Read the model definition and answer for the solid it produces. Units are mm, in the model's axes. A direction names the side the tool comes from. Coordinates: 2 decimals unless noted, no trailing zeros. Write each loop counter-clockwise with the first axis right and the second up, starting at its lowest first coordinate (ties: lowest second). Pieces come first, ordered by that corner, then holes. Notation, with made-up numbers: (18.25, 38.25) - (39.25, 38.25) arc R8 cw to (39.25, 47.25) - close; hole circle Ø9 at (-6.75, 79). An arc over 180 degrees is marked (long way). Use a Markdown table: item, result.
from build123d import *

# Parameters (mm, degrees)
F1_DEPTH = 483.87
F2_R     = 63.5
F3_DEPTH = 142.24
F4_R     = 38.1
F5_DEPTH = 73.66
F6_R     = 127
F7_R     = 127
F8_R     = 127
F9_R     = 127


with BuildPart() as f1:
    # F0 (on Front) → F1 (new body)
    with BuildSketch(Plane.XZ):
        with BuildLine():
            ThreePointArc((-483.137783, 181.369661), (-513.944341, 81.678197), (-449.012806, 0))
            Line((-449.012806, 0), (820.987194, 0))
            Line((820.987194, 0), (820.987194, 48.26))
            Line((820.987194, 48.26), (-449.012806, 48.26))
            ThreePointArc((-449.012806, 48.26), (-469.513207, 97.752345), (-449.012806, 147.244691))
            Line((-449.012806, 147.244691), (0, 596.257497))
            Line((0, 596.257497), (-34.124973, 630.38247))
            Line((-34.124973, 630.38247), (-483.137783, 181.369661))
        make_face()
    extrude(amount=F1_DEPTH)

    # F2 (on face) → F3 (cut)
    with BuildSketch(Plane(origin=(0, 0, 0), x_dir=(1, 0, 0), z_dir=(0, 0, -1))):
        with Locations((8.187194, 241.935)):
            Circle(F2_R)
        with BuildLine():
            ThreePointArc((389.187194, 178.435), (434.088475, 197.033719), (452.687194, 241.935))
            ThreePointArc((452.687194, 241.935), (434.088475, 286.836281), (389.187194, 305.435))
            ThreePointArc((389.187194, 305.435), (325.687194, 241.935), (389.187194, 178.435))
        make_face()
        with BuildLine():
            ThreePointArc((389.187194, 305.435), (434.088475, 286.836281), (452.687194, 241.935))
            ThreePointArc((452.687194, 241.935), (434.088475, 197.033719), (389.187194, 178.435))
            Line((389.187194, 178.435), (643.187194, 178.435))
            ThreePointArc((643.187194, 178.435), (579.687194, 241.935), (643.187194, 305.435))
            Line((643.187194, 305.435), (389.187194, 305.435))
        make_face()
        with BuildLine():
            ThreePointArc((706.687194, 241.935), (688.088475, 286.836281), (643.187194, 305.435))
            ThreePointArc((643.187194, 305.435), (579.687194, 241.935), (643.187194, 178.435))
            ThreePointArc((643.187194, 178.435), (688.088475, 197.033719), (706.687194, 241.935))
        make_face()
    extrude(amount=-F3_DEPTH, mode=Mode.SUBTRACT)

    # F4 (on face) → F5 (cut)
    with BuildSketch(Plane(origin=(-332.253722, 0, 332.253722), x_dir=(0.707107, 0, 0.707107), z_dir=(-0.707107, 0, 0.707107))):
        with Locations((231.117719, -114.3)):
            Circle(F4_R)
        with Locations((231.117719, -369.57)):
            Circle(F4_R)
    extrude(amount=-F5_DEPTH, mode=Mode.SUBTRACT)

    # F6
    f6_edges = [f1.edges().sort_by_distance(p)[0] for p in [
        (-17.062487, -483.87, 613.319983),
    ]]
    fillet(f6_edges, radius=F6_R)

    # F7
    f7_edges = [f1.edges().sort_by_distance(p)[0] for p in [
        (-17.062487, 0, 613.319983),
    ]]
    fillet(f7_edges, radius=F7_R)

    # F8
    f8_edges = [f1.edges().sort_by_distance(p)[0] for p in [
        (820.987194, -483.87, 24.13),
    ]]
    fillet(f8_edges, radius=F8_R)

    # F9
    f9_edges = [f1.edges().sort_by_distance(p)[0] for p in [
        (820.987194, 0, 24.13),
    ]]
    fillet(f9_edges, radius=F9_R)


solid = f1.part
(1) A cutting plane is placed at C-C, the plane y = -432. Write down the section's boundary in (x, z).
Report:
| item | result |
|---|---|
| outline | (-483.14, 181.37) arc R111.76 ccw to (-449.01, 0) - (796.38, 0) - (796.38, 48.26) - (-449.01, 48.26) arc R69.99 cw to (-449.01, 147.24) - (-17.4, 578.86) - (-51.52, 612.98) - close |
(2) Straight lines are drawn through the part: L1, parallel to Z at x = 309.5, y = -218; L2, parallel to Z at x = -386, y = -27; L3, parallel to Z at x = -164, y = -123. For each, find the intervals that lie inside material, in ascending order.
Report:
| item | result |
|---|---|
| L1 | z = 0 to 48.26 |
| L2 | z = 0 to 48.26, 210.26 to 278.51 |
| L3 | z = 0 to 48.26, 432.26 to 438.39 |
(3) Each of these flat-tipped pins is pushed along its axis until it touches: P1, Ø10, axis at y = -171, z = 221, coming from the +X side; P2, Ø2, axis at y = -202, z = 558, coming from the +X side; P3, Ø1, axis at y = -340.5, z = 282.5, coming from the +X side; P4, Ø8, axis at x = 123.5, y = -140, coming from the -Z side. Where does it stop, or does it pass through?
Report:
| item | result |
|---|---|
| P1 | stops at x = -370.26 |
| P2 | stops at x = -37.26 |
| P3 | stops at x = -313.26 |
| P4 | stops at z = 0 |
(4) The mould has two halves that part along X. Classify faces 4 (the flat face through (-48, 0, 31)), 5 (the flat face through (-16.82, -240.33, 613.08)), 6 (the cylindrical face through (-5.578, -179.945, 23.792)): pulls with the +X half, pulls with the -X half, needs draft (parallel to the pull), parting line crosses it, or undercut.
Report:
| item | result |
|---|---|
| face 4 | needs draft |
| face 5 | pulls with the +X half |
| face 6 | undercut |
(5) A cutting plane is placed at A-A, the plane x = 606. Write down the section's boundary in (y, z) (3 decimals).
Report:
| item | result |
|---|---|
| outline | (-483.87, 0) - (-305.435, 0) - (-305.435, 48.26) - (-483.87, 48.26) - close; (-178.435, 0) - (0, 0) - (0, 48.26) - (-178.435, 48.26) - close |
(6) For faces 1 (the flat face through (518, -305.435, 24)), 2 (the flat face through (195, -239, 48.26)), 3 (the flat face through (-255.49, -238.55, 409.02)), determine the directions among +Z, -Z, +X, -X, +Y, -Y from which every point of the face is accessible in a straight line to the end or side of a thin tool.
Report:
| item | result |
|---|---|
| face 1 | +Z, -Z |
| face 2 | +X, +Y, -Y |
| face 3 | +Z, -X, +Y, -Y |
(7) A cutting plane is placed at B-B, the plane x = 36. Write down the section's boundary in (y, z).
Report:
| item | result |
|---|---|
| outline | (-483.87, 0) - (-299.02, 0) - (-299.02, 48.26) - (-483.87, 48.26) - close; (-184.85, 0) - (0, 0) - (0, 48.26) - (-184.85, 48.26) - close |
(8) A cutting plane is placed at D-D, the plane z = 387.5. Write down the section's boundary in (x, y), and give its area (3 significant figures).
Report:
| item | result |
|---|---|
| outline | (-277.01, -483.87) - (-208.76, -483.87) - (-208.76, 0) - (-277.01, 0) - close |
| area | 33,000 mm² |
